```python
from build123d import *

# Parameters (mm, degrees)
SKETCH1_R           = 4
BOSS_EXTRUDE1_DEPTH = 70
SKETCH2_W           = 54
SKETCH2_H           = 49.5
CUT_EXTRUDE1_DEPTH  = 35
HOLE1_AT_2_COUNT    = 2
HOLE1_AT_2_PITCH    = 34


with BuildPart() as part:
    # Sketch1 → Boss-Extrude1 (new body)
    with BuildSketch(Plane.XY):
        with BuildLine():
            Line((-12.5, 22.5), (-12.5, -22.5))
            Line((-12.5, -22.5), (12.5, -22.5))
            Line((12.5, -22.5), (12.5, 22.5))
            ThreePointArc((12.5, 22.5), (0, 35), (-12.5, 22.5))
        make_face()
        with Locations((0, 22.5)):
            Circle(SKETCH1_R, mode=Mode.SUBTRACT)
    extrude(amount=-BOSS_EXTRUDE1_DEPTH)

    # Sketch2 → Cut-Extrude1 (cut, symmetric)
    with BuildSketch(Plane(origin=(12.5, 0, 0), x_dir=(0, 0, -1), z_dir=(1, 0, 0))):
        with Locations((35, 10.25)):
            Rectangle(SKETCH2_W, SKETCH2_H)
    extrude(amount=CUT_EXTRUDE1_DEPTH, both=True, mode=Mode.SUBTRACT)

    # Sketch5 → Hole1 (revolve, cut)
    with BuildSketch(Plane(origin=(0, -14.5, -52), x_dir=(0, 0, 1), z_dir=(1, 0, 0))):
        Polygon((0, 0), (0, 8), (3, 8), (3, 6.201721238), (5, 5), (5, 0), align=None)
    hole1 = revolve(axis=Axis((0, -8.369976101, -52), (0, -1, 0)), mode=Mode.SUBTRACT)

    # Hole1 at 2: Hole1 ×2
    with Locations(*[(0, 0, i * HOLE1_AT_2_PITCH) for i in range(1, HOLE1_AT_2_COUNT)]):
        add(hole1, mode=Mode.SUBTRACT)


solid = part.part
```
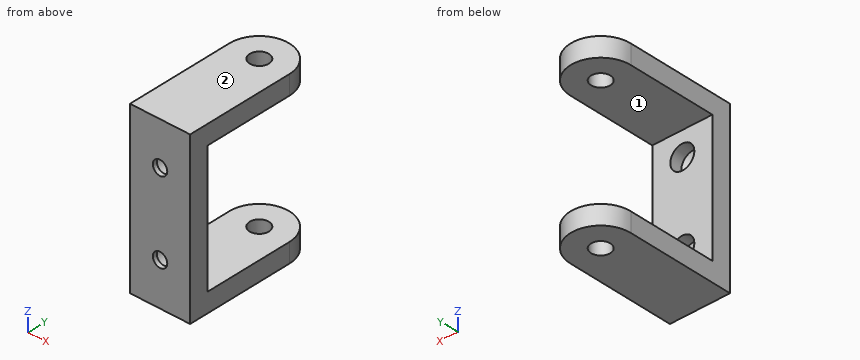
The model under review builds one solid part; all positions refer to its coordinate system, in mm. Face numbers are marked on the shaded views. A direction names the side the tool comes from. Coordinates: 2 decimals unless noted, no trailing zeros. Write each loop counter-clockwise with the first axis right and the second up, starting at its lowest first coordinate (ties: lowest second). Pieces come first, ordered by that corner, then holes. Notation, with made-up numbers: (12.25, 16) -> (49.25, 16) arc R11 ccw to (49.25, 25) -> close; hole circle Ø5 at (86, -4). An arc over 180 degrees is marked (long way). One line per item, written item: value. Start each with the question number.
Q1. Add section A-A, the plane x = 0. Count the separate pieces of the cut face and the enclosed holes in it, then the cut area to 3 significant figures.
Q2. For the marked faces 1 and 2, list the 3-axis set-ups (+Z, -Z, +X, -X, +Y, -Y) from which the entire face can be reached by the end or side of a thin tool; tool diameter is ignored.
Q3. Add section D-D, the plane z = -18. Give the boundary of the cut face in (x, y).
Q4. To check wall thickness, follow probe 1 along Z at (x, y) = (0, -22.1); probe 2 along Z at (x, y) = (5, -8); probe 3 along Z at (x, y) = (0, -15.6). State the ranges of each line that lie inside material, in increasing order.
Q5. Clearance check with flat-ended pins moving along their axes: P1, Ø6, axis at x = 0.5, z = -42.5, coming from the +Y side; P2, Ø3.5, axis at x = 0, z = -52, coming from the +Y side. State where each tip first meets the part, or that it passes through.
Q6. Add section B-B, the plane z = -7. Give the boundary of the cut face in (x, y), then the cut area to 3 significant figures.
Q7. Add section C-C, the plane y = 2. Give the boundary of the cut face in (x, z).
Response:
1. separate pieces: 5
1. enclosed holes: 0
1. area: 1,080 mm²
2. face 1: +X, -X, +Y
2. face 2: +Z, +X, -X, +Y, -Y
3. outline: (-12.5, -22.5) -> (-3, -22.5) -> (-3, -20.7) -> (-5, -19.5) -> (-5, -14.5) -> (-12.5, -14.5) -> close; (3, -22.5) -> (12.5, -22.5) -> (12.5, -14.5) -> (5, -14.5) -> (5, -19.5) -> (3, -20.7) -> close
4. probe 1: -70 to -55, -49 to -21, -15 to 0
4. probe 2: -70 to -62, -8 to 0
4. probe 3: -70 to -57, -47 to -23, -13 to 0
5. P1: y = -14.5
5. P2: through
6. outline: (-12.5, -22.5) -> (12.5, -22.5) -> (12.5, 22.5) arc R12.5 ccw to (-12.5, 22.5) -> close; hole circle Ø8 at (0, 22.5)
6. area: 1,320 mm²
7. outline: (-12.5, -70) -> (12.5, -70) -> (12.5, -62) -> (-12.5, -62) -> close; (-12.5, -8) -> (12.5, -8) -> (12.5, 0) -> (-12.5, 0) -> close
